Verification items for the finished model (mm, model axes). Coordinates: 2 decimals unless noted, no trailing zeros. Write each loop counter-clockwise with the first axis right and the second up, starting at its lowest first coordinate (ties: lowest second). Pieces come first, ordered by that corner, then holes. Notation, with made-up numbers: M -11.75,25.25 L 4.25,25.25 A29 cw 4.25,61.25 Z; hole C 13.25,56 d1. An arc over 180 degrees is marked long. Answer in a Markdown table with one row per item.
Autodesk Inventor part; units mm, degrees
ref_plane "YZ Plane" through (0, 0, 0) normal (1, 0, 0) x (0, 1, 0)
ref_plane "XZ Plane" through (0, 0, 0) normal (0, 1, 0) x (-1, 0, 0)
ref_plane "XY Plane" through (0, 0, 0) normal (0, 0, 1) x (1, 0, 0)
sketch "Эскиз1" plane through (0, 0, 0) normal (0, 1, 0) x (-1, 0, 0)
  circle A0 centre (0, 0) radius 39.5
  circle A1 centre (0, 0) radius 4
  dimension "d0" = 79
  dimension "d3" = 8
extrude "Выдавливание2" add sketch "Эскиз1" along normal blind 4
sketch "Эскиз3" plane through (0, 0, 0) normal (0, -1, 0) x (1, 0, 0)
  circle A0 centre (16.284, 0.1089) radius 4.75
  circle A1 centre (-15.9974, -0.2901) radius 4.75
  circle A2 centre (0, 0) radius 4.5
  dimension "d8" = 9
extrude "Выдавливание3" cut sketch "Эскиз3" against normal blind 4
sketch "Эскиз4" plane through (0, 4, 0) normal (0, 1, 0) x (1, 0, 0)
  circle A0 centre (-27.7164, 11.4805) radius 4 construction
  circle A1 centre (-27.7164, 11.4805) radius 3.15
  point P0 (0, 0)
  dimension "d11" = 6.3
extrude "Выдавливание4" cut sketch "Эскиз4" against normal blind 4
pattern_circular "Круговой массив1" count 4 over 360 about axis through (0, 0, 0) along (0, 1, 0) of "Выдавливание4"
properties part number "Prostavka"
1) Release check for a two-part mould opening along Z. For faces 1 (the face through (-0.59, 1.97, 4.46)), 2 (the face through (-11.619, 2.028, 30.863)), 3 (the face through (-8, 0, 1)), 4 (the face through (29.11, 1.97, -26.7)) record: +Z half, -Z half, draft (parallel to the pull), parting line (faces both ways), or undercut.
Response values:
| item | result |
|---|---|
| face 1 | undercut |
| face 2 | undercut |
| face 3 | draft |
| face 4 | parting line |
2) Sectioned sample at C-C (y = 0.9). Record the cut outline in (x, z).
Response values:
| item | result |
|---|---|
| outline | C 0,0 d79; hole C -27.72,-11.48 d6.3; hole C -16,-0.29 d9.5; hole C -11.48,27.72 d6.3; hole C 0,0 d9; hole C 11.48,-27.72 d6.3; hole C 16.28,0.11 d9.5; hole C 27.72,11.48 d6.3 |
3) Sectioned sample at D-D (z = 20.5). Record the cut outline in (x, y), then the cut area to 3 significant figures.
Response values:
| item | result |
|---|---|
| outline | M -33.76,0 L 33.76,0 L 33.76,4 L -33.76,4 Z |
| area | 270 mm² |
4) Depth check by flat-ended pin: pin 1 (7 mm diameter, centred on x = 27.72, z = 11.48, fed in from +Y); pin 2 (4 mm diameter, centred on x = -11.48, z = 27.72, fed in from -Y); pin 3 (2 mm diameter, centred on y = 3.5, z = 31, fed in from -X). Enter the tip coordinate at first touch or a pass-through.
Response values:
| item | result |
|---|---|
| pin 1 | stops at y = 4 |
| pin 2 | passes through |
| pin 3 | stops at x = -25.7 |
5) Sectioned sample at B-B (z = 12.5). Record the cut outline in (x, y).
Response values:
| item | result |
|---|---|
| outline | M -37.47,0 L 24.74,0 L 24.74,4 L -37.47,4 Z; M 30.7,0 L 37.47,0 L 37.47,4 L 30.7,4 Z |
6) Thickness scan on L1, parallel to Z at x = 0, y = 2.65; L2, parallel to X at y = 1.25, z = -2; L3, parallel to X at y = 1.05, z = 1. Record the ranges inside material, lowest first. Write a range as [from, to].
Response values:
| item | result |
|---|---|
| L1 | z = [-39.5, -4.5], [4.5, 39.5] |
| L2 | x = [-39.45, -20.43], [-11.57, -4.03], [4.03, 12.03], [20.54, 39.45] |
| L3 | x = [-39.49, -20.57], [-11.43, -4.39], [4.39, 11.62], [20.95, 39.49] |
7) Sectioned sample at A-A (x = 0). Record the cut outline in (y, z), then the cut area to 3 significant figures.
Response values:
| item | result |
|---|---|
| outline | M 0,-39.5 L 4,-39.5 L 4,-4.5 L 0,-4.5 Z; M 0,4.5 L 4,4.5 L 4,39.5 L 0,39.5 Z |
| area | 280 mm² |
